The listing builds one solid part. Answer for the finished solid, in the listing's coordinates (mm). A direction names the side the tool comes from. Round coordinates to 2 decimals unless told otherwise and drop trailing zeros. Write each loop counter-clockwise with the first axis right and the second up, starting at its lowest first coordinate (ties: lowest second). Pieces come first, ordered by that corner, then holes. Notation, with made-up numbers: M 55,41.25 L 111,41.25 A7 ccw 111,53.25 Z; hole C -8.5,73.25 d11. An arc over 180 degrees is marked long. Answer as CSV lines item,"result". Start each with the question number.
from build123d import *

# Parameters (mm, degrees)
ESBO_O1_R                = 1.75
RESSALTO_EXTRUS_O1_DEPTH = 4
ESBO_O2_W                = 42
ESBO_O2_H                = 29
ESBO_O2_R                = 1.75
RESSALTO_EXTRUS_O2_DEPTH = 4


with BuildPart() as part:
    # Esboço1 → Ressalto-extrusão1 (new body)
    with BuildSketch(Plane.XY):
        with BuildLine():
            Line((-20.5, -21.5), (-20.5, 21.5))
            Line((-20.5, 21.5), (21.5, 21.5))
            Line((21.5, 21.5), (21.5, 11.5))
            Line((21.5, 11.5), (4.898979486, 11.5))
            ThreePointArc((4.898979486, 11.5), (-9.56053111, 8.052716616), (-10.5, -6.782329983))
            Line((-10.5, -6.782329983), (-10.5, -21.5))
            Line((-10.5, -21.5), (-20.5, -21.5))
        make_face()
        with Locations((-15.5, 15.5)):
            Circle(ESBO_O1_R, mode=Mode.SUBTRACT)
        with Locations((15.5, 15.5)):
            Circle(ESBO_O1_R, mode=Mode.SUBTRACT)
        with Locations((-15.5, -15.5)):
            Circle(ESBO_O1_R, mode=Mode.SUBTRACT)
    extrude(amount=RESSALTO_EXTRUS_O1_DEPTH)

    # Esboço2 → Ressalto-extrusão2 (add)
    with BuildSketch(Plane(origin=(0, 21.5, 0), x_dir=(1, 0, 0), z_dir=(0, 1, 0))):
        with Locations((0.5, 0.5)):
            Rectangle(ESBO_O2_W, ESBO_O2_H)
        with Locations(Location((-14.5, -9, 0), (0, 0, 270))):
            Circle(ESBO_O2_R, mode=Mode.SUBTRACT)
        with Locations(Location((15.5, -9, 0), (0, 0, 270))):
            Circle(ESBO_O2_R, mode=Mode.SUBTRACT)
    extrude(amount=RESSALTO_EXTRUS_O2_DEPTH)


solid = part.part
Q1. Find section D-D (x = -15.5). Determine the outline of the cut face in (y, z), plus the area to 3 significant figures.
Q2. The mould has two halves that part along X. Classify faces 1 (the face through (-14.6, 17, 2)), 2 (the face through (0, 23, -15)), 3 (the face through (-20.5, 9, 1)): +X half, -X half, draft (parallel to the pull), parting line (faces both ways), or undercut.
Q3. Find section A-A (y = -15.5). Determine the outline of the cut face in (x, z).
Q4. Straight lines are drawn through the part: L1, parallel to Y at x = -15.5, z = 1.5; L2, parallel to X at y = 23.95, z = 9; L3, parallel to Y at x = 15.5, z = 3.1. For each, find the intervals that lie inside material, in ascending order.
Q5. Find section C-C (z = 1.75). Determine the outline of the cut face in (x, y).
Q6. Each of these flat-tipped pins is pushed along its axis until it touches: P1, Ø5, axis at x = -5, y = 10, coming from the +Z side; P2, Ø5, axis at x = -5, z = 8, coming from the -Y side; P3, Ø4, axis at x = -15.5, y = 15.5, coming from the -Z side. Where does it stop, or does it pass through?
Q7. Find section B-B (y = 15.5). Determine the outline of the cut face in (x, z), plus the area to 3 significant figures.
Q8. For faces 4 (the face through (-10.5, -14, 2)), 5 (the face through (-9, 10, 4)), 6 (the face through (-9, 10, 0)), 7 (the face through (-9.415, 8.222, 1.972)), 8 (the face through (17.235, 23.472, 8.772)), determine the directions among +Z, -Z, +X, -X, +Y, -Y from which every point of the face is accessible in a straight line to the end or side of a thin tool.
Reported:
1,outline,"M -21.5,0 L -17.25,0 L -17.25,4 L -21.5,4 Z; M -13.75,0 L 13.75,0 L 13.75,4 L -13.75,4 Z; M 17.25,0 L 21.5,0 L 21.5,-15 L 25.5,-15 L 25.5,7.56 L 21.5,7.56 L 21.5,4 L 17.25,4 Z; M 21.5,10.44 L 25.5,10.44 L 25.5,14 L 21.5,14 Z"
1,area,"249 mm2"
2,face 1,"undercut"
2,face 2,"draft"
2,face 3,"-X half"
3,outline,"M -20.5,0 L -17.25,0 L -17.25,4 L -20.5,4 Z; M -13.75,0 L -10.5,0 L -10.5,4 L -13.75,4 Z"
4,L1,"y = -21.5 to -17.25, -13.75 to 13.75, 17.25 to 25.5"
4,L2,"x = -20.5 to -16.25, -12.75 to 13.75, 17.25 to 21.5"
4,L3,"y = 11.5 to 13.75, 17.25 to 25.5"
5,outline,"M -20.5,-21.5 L -10.5,-21.5 L -10.5,-6.78 A12.5 cw 4.9,11.5 L 21.5,11.5 L 21.5,25.5 L -20.5,25.5 Z; hole C -15.5,-15.5 d3.5; hole C -15.5,15.5 d3.5; hole C 15.5,15.5 d3.5"
6,P1,"stops at z = 4"
6,P2,"stops at y = 21.5"
6,P3,"stops at z = 0"
7,outline,"M -20.5,0 L -17.25,0 L -17.25,4 L -20.5,4 Z; M -13.75,0 L 13.75,0 L 13.75,4 L -13.75,4 Z; M 17.25,0 L 21.5,0 L 21.5,4 L 17.25,4 Z"
7,area,"140 mm2"
8,face 4,"+Z, -Z, +X, -Y"
8,face 5,"+Z, +X, -X, -Y"
8,face 6,"-Z, +X, -X, -Y"
8,face 7,"+Z, -Z"
8,face 8,"+Y, -Y"
